Can you work these out from the model? Positions are in its coordinate system, mm. A direction names the side the tool comes from. Coordinates: 2 decimals unless noted, no trailing zeros. Order: outer loops, then holes, each group sorted by start corner. A loop starts at its lowest first (then second) coordinate and runs counter-clockwise, first axis right, second up. Notation, with made-up numbers: (-32, 69) -> (1, 69) arc R37 cw to (1, 108) -> close; hole circle Ø2 at (71.5, -18.75). An arc over 180 degrees is marked (long way). Write item = value, one per line. Start each with the question number.
from build123d import *

# Parameters (mm, degrees)
F0_W     = 50.8
F0_H     = 50.8
F1_DEPTH = 25.4


with BuildPart() as f1:
    # F0 (on Front) → F1 (new body)
    with BuildSketch(Plane.XZ):
        Polygon((-10.1240915534, 65.3393898586), (-48.9609619458, 32.592825182), (-33.8989773116, 32.592825182), (-10.1240915534, 52.6393898586), align=None)
        Polygon((-33.8989773116, 32.592825182), (-48.9609619458, 32.592825182), (-48.9609619458, 19.892825182), align=None)
        Polygon((1.8390380542, 32.592825182), (-33.8989773116, 32.592825182), (-48.9609619458, 19.892825182), (1.8390380542, 19.892825182), align=None)
        Polygon((40.6759084466, 65.3393898586), (-10.1240915534, 65.3393898586), (-10.1240915534, 52.6393898586), (25.6139238124, 52.6393898586), align=None)
        with Locations((15.2759084466, 90.7393898586)):
            Rectangle(F0_W, F0_H)
        Polygon((25.6139238124, 52.6393898586), (1.8390380542, 32.592825182), (1.8390380542, 19.892825182), (40.6759084466, 52.6393898586), align=None)
        Polygon((40.6759084466, 52.6393898586), (40.6759084466, 65.3393898586), (25.6139238124, 52.6393898586), align=None)
        Polygon((-10.1240915534, 52.6393898586), (-33.8989773116, 32.592825182), (1.8390380542, 32.592825182), (25.6139238124, 52.6393898586), align=None)
    extrude(amount=-F1_DEPTH)


solid = f1.part
(1) For faces 1 (the face through (-10.124, 13, 90)), 2 (the face through (5, 25.4, 69)), which set-ups out of +Z, -Z, +X, -X, +Y, -Y let a thin tool reach every point of the face, with its end or its side?
(2) Imagine slicing it at B-B (z = 107). Write out the boundary of the cut face in (x, y).
(3) If I drill on L1, parallel to X at y = 17, z = 100.5; L2, parallel to Z at x = 26, y = 22; L3, parallel to Z at x = -11.5, y = 23, over which ranges is the centre line in solid material (lowest first)? Write a range as from..to.
(4) Imagine slicing it at A-A (y = 11). Write out the boundary of the cut face in (x, z), plus the area to 3 significant figures.
(5) For P1, Ø8, axis at y = 22.5, z = 63.5, coming from the -X side; P2, Ø6, axis at y = 3, z = 102, coming from the -X side; P3, Ø3, axis at x = -37, y = 18.5, coming from the +Z side; P4, Ø3, axis at x = -20.5, z = 41.5, coming from the -Y side, each with a flat end and sliding along its axis, tell me the tip position at first contact or that it passes through.
(6) Imagine slicing it at C-C (x = 34). Write out the boundary of the cut face in (y, z), plus the area to 3 significant figures.
Result set:
q1.face_1 = +Z, -X, +Y, -Y
q1.face_2 = +Z, -Z, +X, -X, +Y
q2.outline = (-10.12, 0) -> (40.68, 0) -> (40.68, 25.4) -> (-10.12, 25.4) -> close
q3.L1 = -10.12..40.68
q3.L2 = 40.26..116.14
q3.L3 = 19.89..64.18
q4.outline = (-48.96, 19.89) -> (1.84, 19.89) -> (40.68, 52.64) -> (40.68, 116.14) -> (-10.12, 116.14) -> (-10.12, 65.34) -> (-48.96, 32.59) -> close
q4.area = 5,380 mm2
q5.P1 = -17.05
q5.P2 = -10.12
q5.P3 = 43.94
q5.P4 = 0
q6.outline = (0, 47.01) -> (25.4, 47.01) -> (25.4, 116.14) -> (0, 116.14) -> close
q6.area = 1,760 mm2
